Can you work these out from the drawing? Everything is in mm from the part's minimum corner. A direction names the side the tool comes from. Coordinates: 2 decimals unless noted, no trailing zeros. Order: outer loops, then holes, each group sorted by start corner. A loop starts at its lowest first (then second) coordinate and runs counter-clockwise, first axis right, second up. Notation, with made-up numbers: (78, 10.5) -> (137, 10.5) arc R19 ccw to (137, 18.5) -> close; hole circle Ø5 at (8.5, 2.25). An arc over 180 degrees is marked (long way). Return JSON: item names as keys, results as strings. Group by question number.
1) For the marked faces 1 and 2, which set-ups out of +Z, -Z, +X, -X, +Y, -Y let a thin tool reach every point of the face, with its end or its side?
2) If we section it at B-B, the plane z = 2: Please give me the cut outline in (x, y).
3) Thinking about a two-plate mould opening in X: for the marked faces 3, 4 and 5, which applies, +X half, -X half, draft (parallel to the pull), parting line (faces both ways), or undercut?
4) If I drill on probe 1 along X at (y, z) = (4.55, 5.5); probe 2 along X at (y, z) = (4.9, 4.5); probe 3 along Y at (x, z) = (9, 0.5), over which ranges is the centre line in solid material (lowest first)? Write a range as from..to.
5) If we section it at A-A, the plane y = 4.5: Please give me the cut outline in (x, z), then the cut area to 3 significant figures.
6) For pin 1 (1.5 mm diameter, centred on x = 8, z = 9, fed in from +Y), with a flat end and sliding along its axis, tell me the tip position at first contact or that it passes through.
7) If we section it at D-D, the plane y = 2.3: Please give me the cut outline in (x, z).
8) If we section it at C-C, the plane x = 4: Please give me the cut outline in (y, z), then the cut area to 3 significant figures.
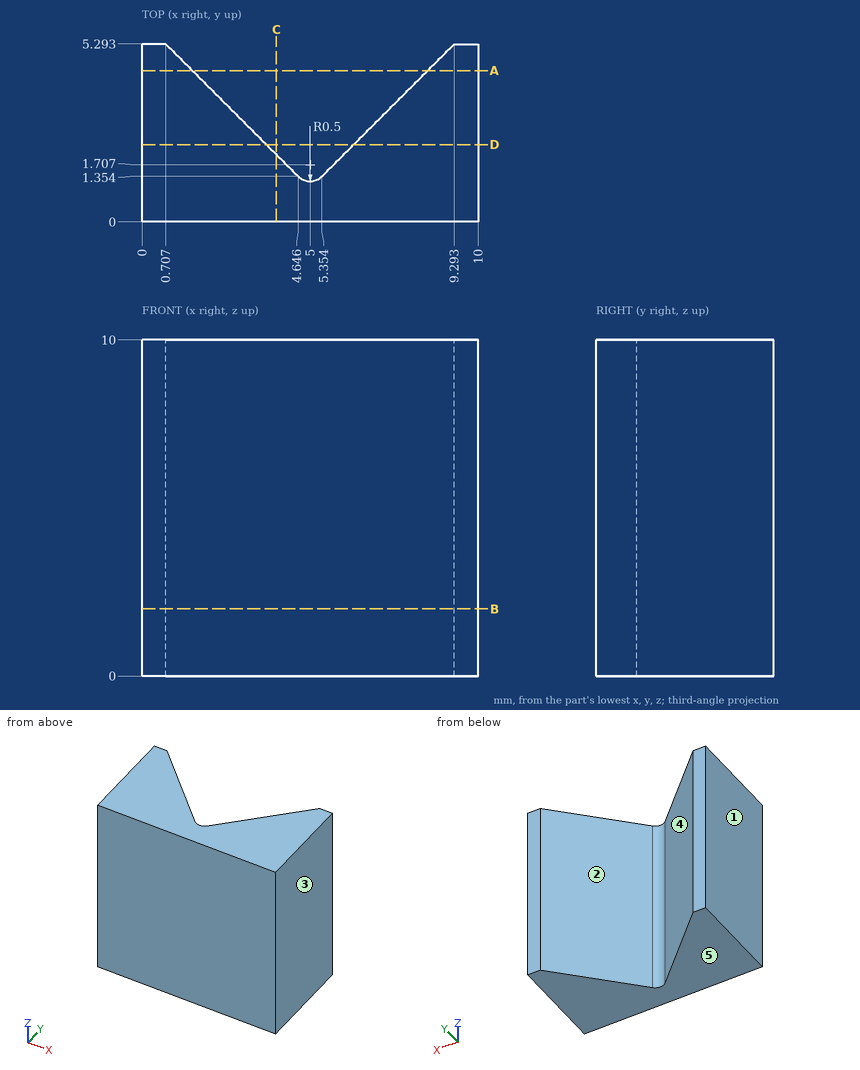
Result sheet:
{
 "1": {"face 1": "+Z, -Z, -X, +Y, -Y", "face 2": "+Z, -Z, +Y"},
 "2": {"outline": "(0, 0) -> (10, 0) -> (10, 5.29) -> (9.29, 5.29) -> (5.35, 1.35) arc R0.5 cw to (4.65, 1.35) -> (0.71, 5.29) -> (0, 5.29) -> close"},
 "3": {"face 3": "+X half", "face 4": "undercut", "face 5": "draft"},
 "4": {"probe 1": "x = 0..1.45, 8.55..10", "probe 2": "x = 0..1.1, 8.9..10", "probe 3": "y = 0..5"},
 "5": {"outline": "(0, 0) -> (1.5, 0) -> (1.5, 10) -> (0, 10) -> close; (8.5, 0) -> (10, 0) -> (10, 10) -> (8.5, 10) -> close", "area": "30.0 mm2"},
 "6": {"pin 1": "stops at y = 4.75"},
 "7": {"outline": "(0, 0) -> (3.7, 0) -> (3.7, 10) -> (0, 10) -> close; (6.3, 0) -> (10, 0) -> (10, 10) -> (6.3, 10) -> close"},
 "8": {"outline": "(0, 0) -> (2, 0) -> (2, 10) -> (0, 10) -> close", "area": "20.0 mm2"}
}
